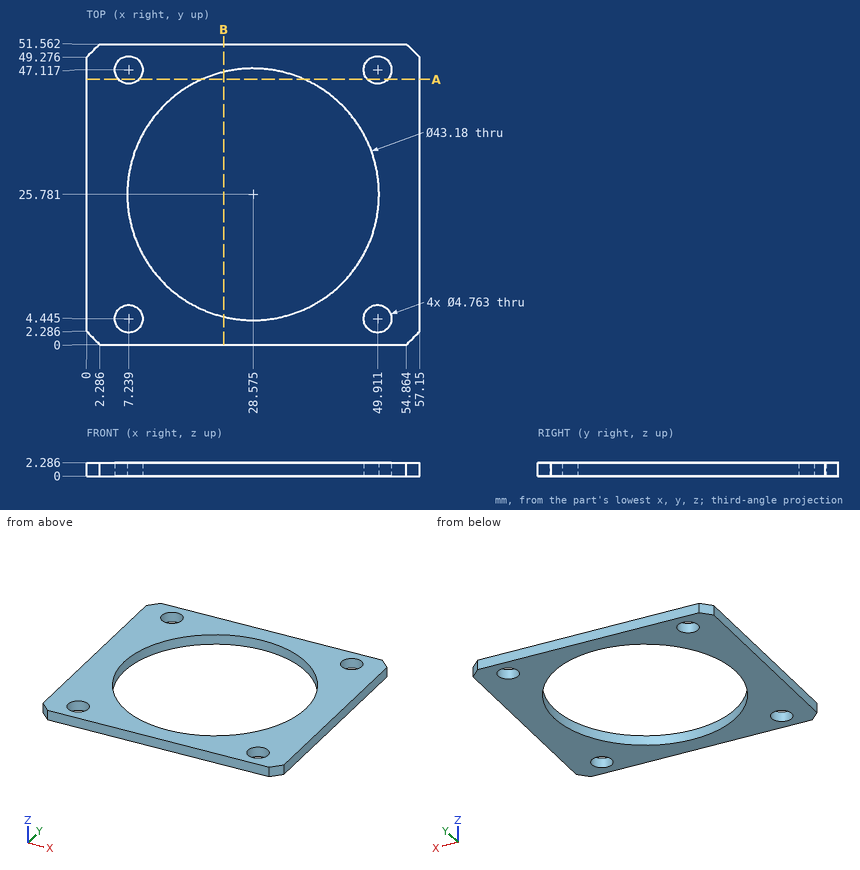
Geometry: see drawing. Coordinates: mm, zero at the bounding-box minimum. Round coordinates to 2 decimals unless told otherwise and drop trailing zeros. Loops run counter-clockwise (first coordinate to the right, second up) from the corner with the lowest first, then second, coordinate; pieces in that order, holes last. Notation, with made-up numbers: (77.5, 53.25) -> (106.5, 53.25) arc R27 ccw to (106.5, 73.25) -> close; hole circle Ø2 at (-40, 10). An arc over 180 degrees is marked (long way). One line per question, with ' | ' between items. Start each with the question number.
1. Section A-A on y = 45.5. Count the separate pieces of the cut face and the enclosed holes in it.
2. Section B-B on x = 23.5. Output: boundary loops of the cut face in (y, z) (1 decimal).
3. Line query: line 1 along X through (y, z) = (47.5, 1.75); line 2 along X through (y, z) = (24.5, 1.1); line 3 along X through (y, z) = (27.5, 2). Output: solid intervals per line, ascending. Write a range as [from, to].
Returned:
1) separate pieces: 4 | enclosed holes: 0
2) outline: (0, 0) -> (4.8, 0) -> (4.8, 2.3) -> (0, 2.3) -> close; (46.8, 0) -> (51.6, 0) -> (51.6, 2.3) -> (46.8, 2.3) -> close
3) line 1: x = [0, 4.89], [9.59, 47.56], [52.26, 57.15] | line 2: x = [0, 7.02], [50.13, 57.15] | line 3: x = [0, 7.05], [50.1, 57.15]
